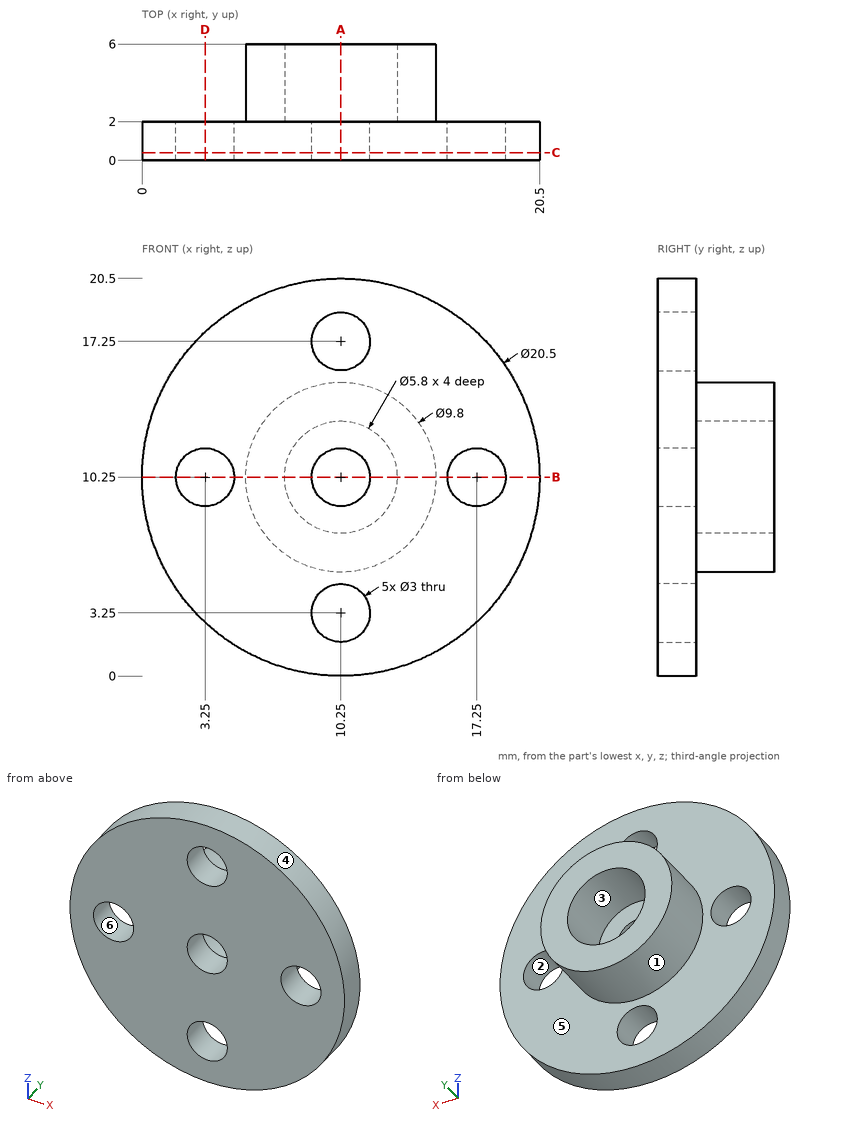
Geometry check sheet. Reference: drawing and pictorial views, mm from the part's lowest x, y, z. A direction names the side the tool comes from. Give positions to 0.01 mm unless a question says otherwise; leave off trailing zeros. Order: outer loops, then holes, each group sorted by start corner. A loop starts at its lowest first (then second) coordinate and runs counter-clockwise, first axis right, second up. Notation, with made-up numbers: M 76.5,24.5 L 91.5,24.5 A19 cw 91.5,41.5 Z; hole C 11.5,43.5 d9. An arc over 180 degrees is marked long. Answer as a JSON object with one key per item and string values. Group by question number.
1) Depth check by flat-ended pin: pin 1 Ø1 at (x, z) = (5.5, 14.5) entering from -Y; pin 2 Ø3 at (x, y) = (4.5, 4.5) entering from -Z; pin 3 Ø1.7 at (x, z) = (10, 9) entering from +Y; pin 4 Ø2 at (x, y) = (5, 5) entering from +Z. Enter the tip coordinate at first touch or a pass-through.
2) Cross-section at D-D (x = 3.25). Enter the section's corners in (y, z), then the cut area to 4 significant figures.
3) Access from +Z, -Z, +X, -X, +Y, -Y to the whole of each face (thin tool, end or side, straight path). Record for the marked faces 1 and 2.
4) Mould release check, pull along X, two halves, no side actions. Record for the marked faces 3, 4, 5 and 6: released by +X, released by -X, zero draft, split by the parting line, or undercut.
5) Scan lines: line 1 along X through (y, z) = (0.9, 10.25); line 2 along X through (y, z) = (4.7, 10.25); line 3 along Y through (x, z) = (1.25, 10.25). Record each from-to range of solid material in increasing order. Write a range as [from, to].
6) Cross-section at A-A (x = 10.25). Enter the section's corners in (y, z).
7) Cross-section at B-B (z = 10.25). Enter the section's corners in (x, y).
8) Cross-section at C-C (y = 0.4). Enter the section's corners in (x, z), then the cut area to 3 significant figures.
Result sheet:
{
 "1": {"pin 1": "stops at y = 0", "pin 2": "stops at z = 7.81", "pin 3": "stops at y = 2", "pin 4": "stops at z = 12.69"},
 "2": {"outline": "M 0,2.76 L 2,2.76 L 2,8.75 L 0,8.75 Z; M 0,11.75 L 2,11.75 L 2,17.74 L 0,17.74 Z", "area": "23.95 mm2"},
 "3": {"face 1": "+Y", "face 2": "+Y, -Y"},
 "4": {"face 3": "undercut", "face 4": "split by the parting line", "face 5": "zero draft", "face 6": "undercut"},
 "5": {"line 1": "x = [0, 1.75], [4.75, 8.75], [11.75, 15.75], [18.75, 20.5]", "line 2": "x = [5.35, 7.35], [13.15, 15.15]", "line 3": "y = [0, 2]"},
 "6": {"outline": "M 0,0 L 2,0 L 2,1.75 L 0,1.75 Z; M 0,4.75 L 2,4.75 L 2,5.35 L 6,5.35 L 6,7.35 L 2,7.35 L 2,8.75 L 0,8.75 Z; M 0,11.75 L 2,11.75 L 2,13.15 L 6,13.15 L 6,15.15 L 2,15.15 L 2,15.75 L 0,15.75 Z; M 0,18.75 L 2,18.75 L 2,20.5 L 0,20.5 Z"},
 "7": {"outline": "M 0,0 L 1.75,0 L 1.75,2 L 0,2 Z; M 4.75,0 L 8.75,0 L 8.75,2 L 7.35,2 L 7.35,6 L 5.35,6 L 5.35,2 L 4.75,2 Z; M 11.75,0 L 15.75,0 L 15.75,2 L 15.15,2 L 15.15,6 L 13.15,6 L 13.15,2 L 11.75,2 Z; M 18.75,0 L 20.5,0 L 20.5,2 L 18.75,2 Z"},
 "8": {"outline": "C 10.25,10.25 d20.5; hole C 3.25,10.25 d3; hole C 10.25,3.25 d3; hole C 10.25,10.25 d3; hole C 10.25,17.25 d3; hole C 17.25,10.25 d3", "area": "295 mm2"}
}
